```python
from build123d import *

# Parameters (mm, degrees)
SKETCH_1_R               = 10.5
SKETCH_1_R_2             = 9.5
EXTRUDE_1_DEPTH          = 40
SKETCH_2_R               = 10.5
EXTRUDE_2_DEPTH          = 1
SKETCH_3_R               = 0.492995
CUT_EXTRUDE_1_DEPTH      = 1
EXTRUDE_START            = 40
SKETCH_6_R               = 10
SKETCH_6_R_2             = 8
EXTRUDE_3_DEPTH          = 1
SKETCH_5_W               = 2
SKETCH_5_H               = 1.2
EXTRUDE_4_DEPTH          = 2
PATTERN_CIRCULAR_1_COUNT = 4


with BuildPart() as part:
    # ｽｹｯﾁ1 → ﾎﾞｽ - 押し出し1 (new body)
    with BuildSketch(Plane.XY):
        Circle(SKETCH_1_R)
        Circle(SKETCH_1_R_2, mode=Mode.SUBTRACT)
    extrude(amount=EXTRUDE_1_DEPTH)

    # ｽｹｯﾁ2 → ﾎﾞｽ - 押し出し2 (add)
    with BuildSketch(Plane.XY):
        Circle(SKETCH_2_R)
    extrude(amount=EXTRUDE_2_DEPTH)

    # ｽｹｯﾁ3 → ｶｯﾄ - 押し出し1 (cut)
    with BuildSketch(Plane.XY):
        with Locations((4.413132646, 3.597662483)):
            Circle(SKETCH_3_R)
    extrude(amount=CUT_EXTRUDE_1_DEPTH, mode=Mode.SUBTRACT)

    # ｽｹｯﾁ6 → ﾎﾞｽ - 押し出し3 (add)
    with BuildSketch(Plane.XY.offset(EXTRUDE_START)):
        Circle(SKETCH_6_R)
        Circle(SKETCH_6_R_2, mode=Mode.SUBTRACT)
    extrude(amount=-EXTRUDE_3_DEPTH)

    # ｽｹｯﾁ5 → ﾎﾞｽ - 押し出し4 (add)
    with BuildSketch(Plane.XY.offset(40)):
        with Locations((7.5, 0)):
            Rectangle(SKETCH_5_W, SKETCH_5_H)
        with Locations((10.48172138, -0.010967172)):
            Rectangle(SKETCH_5_W, SKETCH_5_H)
    extrude_4 = extrude(amount=-EXTRUDE_4_DEPTH)

    # 円形ﾊﾟﾀｰﾝ1: ﾎﾞｽ - 押し出し4 ×4 about axis
    pattern_circular_1_axis = Axis((0, 0, 0), (0, 0, 1))
    for i in range(1, PATTERN_CIRCULAR_1_COUNT):
        add(extrude_4.rotate(pattern_circular_1_axis, i * 360 / PATTERN_CIRCULAR_1_COUNT))


solid = part.part
```
Check sheet for the modelled part. Datum: model origin and axes. Units: mm. A direction names the side the tool comes from. Round coordinates to 2 decimals unless told otherwise and drop trailing zeros. Loops run counter-clockwise (first coordinate to the right, second up) from the corner with the lowest first, then second, coordinate; pieces in that order, holes last. Notation, with made-up numbers: (27.5, 15) - (56.5, 15) arc R29 cw to (56.5, 41) - close; hole circle Ø8 at (-30.5, 24.5). An arc over 180 degrees is marked (long way). Write item = value, one per line. Start each with the question number.
Q1. Release check for a two-part mould opening along Z. For faces 1 (the face through (0, -8.5, 38.5)), 2 (the face through (0, -7, 40)), 3 (the face through (0, -7, 38)), 4 (the face through (-0.589, 11, 39)) record: pulls with the +Z half, pulls with the -Z half, needs draft (parallel to the pull), parting line crosses it, or undercut.
Q2. Access from +Z, -Z, +X, -X, +Y, -Y to the whole of each face (thin tool, end or side, straight path). Record for faces 5 (the face through (-11, -0.589, 39)), 6 (the face through (-8.5, 0, 38.5)), 7 (the face through (-11, 0.611, 39)).
Q3. Depth check by flat-ended pin: P1, Ø1.6, axis at x = -7.5, z = 39, coming from the +Y side; P2, Ø2, axis at y = 7.5, z = 34.5, coming from the +X side; P3, Ø8, axis at y = -1, z = 32.5, coming from the +X side. Enter the tip coordinate at first touch or a pass-through.
Q4. Section check D-D (z = 28). Record the boundary of the cut face in (x, y), plus the area to 3 significant figures.
Q5. Section check C-C (y = -7). Record the boundary of the cut face in (x, z), plus the area to 3 significant figures.
Q6. Thickness scan on L1, parallel to X at y = 0, z = 26; L2, parallel to Z at x = 8.5, y = 1.5; L3, parallel to Z at x = -3.5, y = 4.75. Record the ranges inside material, lowest first.
Derived:
q1.face_1 = undercut
q1.face_2 = pulls with the +Z half
q1.face_3 = undercut
q1.face_4 = needs draft
q2.face_5 = +Z, -Z, -X, -Y
q2.face_6 = none
q2.face_7 = +Z, -Z, -X, +Y
q3.P1 = 8.08
q3.P2 = 8.25
q3.P3 = 10.5
q4.outline = circle Ø21 at (0, 0); hole circle Ø19 at (0, 0)
q4.area = 62.8 mm^2
q5.outline = (-7.83, 0) - (7.83, 0) - (7.83, 40) - (3.87, 40) - (3.87, 39) - (6.42, 39) - (6.42, 1) - (-6.42, 1) - (-6.42, 39) - (-3.87, 39) - (-3.87, 40) - (-7.83, 40) - close; (-0.6, 38) - (0.6, 38) - (0.6, 40) - (-0.6, 40) - close
q5.area = 133 mm^2
q6.L1 = -10.5 to -9.5, 9.5 to 10.5
q6.L2 = 0 to 1, 39 to 40
q6.L3 = 0 to 1
